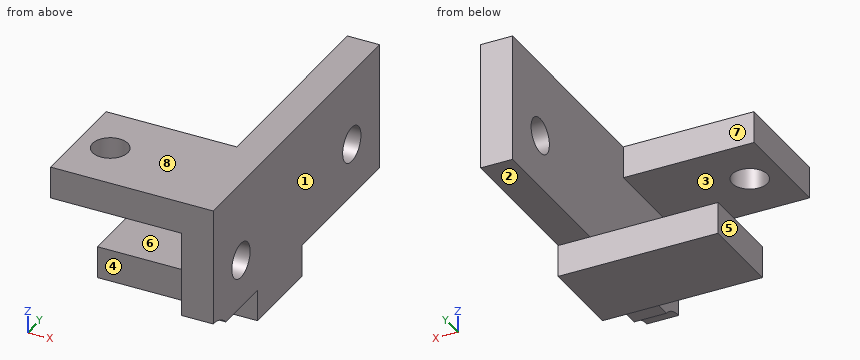
from build123d import *

# Parameters (mm, degrees)
SKETCH_1_W          = 12.25
SKETCH_1_H          = 10
SKETCH_1_R          = 1.65
EXTRUDE_3_DEPTH     = 3
SKETCH_3_W          = 3
SKETCH_3_H          = 10
EXTRUDE_4_DEPTH     = 14
SKETCH_4_R          = 1.65
CUT_EXTRUDE_1_DEPTH = 10
SKETCH_6_W          = 14
SKETCH_6_H          = 20
SKETCH_6_R          = 1.65
EXTRUDE_5_DEPTH     = 3
CUT_EXTRUDE_2_DEPTH = 3
CUT_EXTRUDE_3_REACH = 33.282
SKETCH_8_W          = 2
SKETCH_8_H          = 27.763932023
SKETCH_9_W          = 3
SKETCH_9_H          = 8
EXTRUDE_6_DEPTH     = 15


with BuildPart() as part:
    # 草图1 → 凸台-拉伸3 (new body)
    with BuildSketch(Plane.XY):
        with Locations((3.125, 0)):
            Rectangle(SKETCH_1_W, SKETCH_1_H)
        Circle(SKETCH_1_R, mode=Mode.SUBTRACT)
    extrude(amount=EXTRUDE_3_DEPTH)

    # 草图3 → 凸台-拉伸4 (add)
    with BuildSketch(Plane.XY.offset(3)):
        with Locations((10.75, 0)):
            Rectangle(SKETCH_3_W, SKETCH_3_H)
    extrude(amount=-EXTRUDE_4_DEPTH)

    # 草图4 → 切除-拉伸1 (cut)
    with BuildSketch(Plane(origin=(12.25, 0, 0), x_dir=(0, 0, -1), z_dir=(1, 0, 0))):
        with Locations(Location((4.5, 0, 0), (0, 0, 90))):
            Circle(SKETCH_4_R)
    extrude(amount=-CUT_EXTRUDE_1_DEPTH, mode=Mode.SUBTRACT)

    # 草图6 → 凸台-拉伸5 (add)
    with BuildSketch(Plane(origin=(12.25, 0, 0), x_dir=(0, 0, -1), z_dir=(1, 0, 0))):
        with Locations((4, 15)):
            Rectangle(SKETCH_6_W, SKETCH_6_H)
        with Locations(Location((4, 20, 0), (0, 0, 90))):
            Circle(SKETCH_6_R, mode=Mode.SUBTRACT)
    extrude(amount=-EXTRUDE_5_DEPTH)

    # 草图7 → 切除-拉伸2 (cut)
    with BuildSketch(Plane(origin=(12.25, 0, 0), x_dir=(0, 0, -1), z_dir=(1, 0, 0))):
        with BuildLine():
            Line((8, -5), (11, -5))
            Line((11, -5), (11, -2))
            ThreePointArc((11, -2), (8.878679656, -2.878679656), (8, -5))
        make_face()
    extrude(amount=-CUT_EXTRUDE_2_DEPTH, mode=Mode.SUBTRACT)

    # 草图8 → 切除-拉伸3 (cut, up to next)
    with BuildSketch(Plane(origin=(12.25, 0, 0), x_dir=(0, 0, -1), z_dir=(1, 0, 0)), mode=Mode.PRIVATE) as cut_extrude_3_sk1:
        with Locations((10, 11.118033989)):
            Rectangle(SKETCH_8_W, SKETCH_8_H)
    cut_extrude_3_tool1 = extrude(cut_extrude_3_sk1.sketch, amount=-CUT_EXTRUDE_3_REACH, mode=Mode.PRIVATE) & part.part
    add(cut_extrude_3_tool1.solids().sort_by_distance((12.25, 11.118034, -10))[0], mode=Mode.SUBTRACT)

    # 草图9 → 凸台-拉伸6 (add)
    with BuildSketch(Plane(origin=(12.25, 0, 0), x_dir=(0, 0, -1), z_dir=(1, 0, 0))):
        with Locations((10.5, 7)):
            Rectangle(SKETCH_9_W, SKETCH_9_H)
    extrude(amount=-EXTRUDE_6_DEPTH)


solid = part.part
The listing builds one solid part. Answer for the finished solid, in the listing's coordinates (mm). Face numbers are marked on the shaded views. A direction names the side the tool comes from. Coordinates: 2 decimals unless noted, no trailing zeros. Write each loop counter-clockwise with the first axis right and the second up, starting at its lowest first coordinate (ties: lowest second). Pieces come first, ordered by that corner, then holes. Notation, with made-up numbers: (50.25, 37.25) - (106.25, 37.25) arc R19 cw to (106.25, 42.25) - close; hole circle Ø1 at (29, 76). An arc over 180 degrees is marked (long way). Put each result on its own line as item: value.
1. The part is cut by section B-B on y = 20. Give the vertices of the cut face in (x, z), plus the area to 3 significant figures.
Answer sheet:
outline: (9.25, -9) - (12.25, -9) - (12.25, -5.65) - (9.25, -5.65) - close; (9.25, -2.35) - (12.25, -2.35) - (12.25, 3) - (9.25, 3) - close
area: 26.1 mm^2
2. The part is cut by section C-C on x = 0. Give the vertices of the cut face in (y, z), plus the area to 3 significant figures.
Answer sheet:
outline: (-5, 0) - (-1.65, 0) - (-1.65, 3) - (-5, 3) - close; (1.65, 0) - (5, 0) - (5, 3) - (1.65, 3) - close; (3, -12) - (11, -12) - (11, -9) - (3, -9) - close
area: 44.1 mm^2
3. The part is cut by section D-D on z = -4.5. Give the vertices of the cut face in (x, y).
Answer sheet:
outline: (9.25, -5) - (12.25, -5) - (12.25, -1.65) - (9.25, -1.65) - close; (9.25, 1.65) - (12.25, 1.65) - (12.25, 18.43) - (9.25, 18.43) - close; (9.25, 21.57) - (12.25, 21.57) - (12.25, 25) - (9.25, 25) - close
4. The part is cut by section A-A on x = 8.25. Give the vertices of the cut face in (y, z), plus the area to 3 significant figures.
Answer sheet:
outline: (-5, 0) - (5, 0) - (5, 3) - (-5, 3) - close; (3, -12) - (11, -12) - (11, -9) - (3, -9) - close
area: 54.0 mm^2
5. Determine the mould class of the marked faces 6, 7 and 8 for opening direction Z: pulls with the +Z half, pulls with the -Z half, needs draft (parallel to the pull), parting line crosses it, or undercut.
Answer sheet:
face 6: undercut
face 7: needs draft
face 8: pulls with the +Z half
6. Flat-ended cylindrical pins translate along their axes: pin 1 Ø1.5 at (y, z) = (16, -2) entering from -X; pin 2 Ø1.5 at (x, z) = (6.5, -10) entering from -Y; pin 3 Ø1.5 at (x, z) = (5.5, -10) entering from +Y. Find the tip coordinate at first contact, or state that the pin passes through.
Answer sheet:
pin 1: stops at x = 9.25
pin 2: stops at y = 3
pin 3: stops at y = 11
7. A tool of negligible diameter and unlimited length cuts with its end or side. For the marked faces 1, 2, 3, 4 and 5, from which of +Z, -Z, +X, -X, +Y, -Y can it reach the whole face along a straight path? Write none if from no direction.
Answer sheet:
face 1: +Z, -Z, +X, +Y, -Y
face 2: -Z, +X, -X, +Y
face 3: -X, +Y, -Y
face 4: -Z, +X, -X, -Y
face 5: -Z, -X, +Y, -Y
8. Find the intervals of material crossed by line 1 along Z through (x, y) = (10.95, 0); line 2 along Z through (x, y) = (-1.75, 0); line 3 along X through (y, z) = (21.5, -2.75), in increasing order. Write a range as from..to.
Answer sheet:
line 1: z = -9..-6.15, -2.85..3
line 2: z = 0..3
line 3: x = 9.25..12.25
